from build123d import *

# Parameters (mm, degrees)
SKETCH_1_W          = 13
SKETCH_1_H          = 26
EXTRUDE_1_DEPTH     = 5.57372
SKETCH_2_W          = 13
SKETCH_2_H          = 3
EXTRUDE_2_DEPTH     = 9.8
SKETCH_4_R          = 1
CUT_EXTRUDE_1_DEPTH = 14
CHAMFER_2_SIZE      = 0.8
CHAMFER_2_SIZE2     = 1.385640646
SKETCH_5_R          = 1
EXTRUDE_3_DEPTH     = 13
SKETCH_6_R          = 1
CUT_EXTRUDE_2_DEPTH = 14


with BuildPart() as part:
    # ｽｹｯﾁ1 → ﾎﾞｽ - 押し出し1 (new body)
    with BuildSketch(Plane(origin=(0, 0, 0), x_dir=(1, 0, 0), z_dir=(0, 1, 0))):
        with Locations((6.5, 13)):
            Rectangle(SKETCH_1_W, SKETCH_1_H)
    extrude(amount=EXTRUDE_1_DEPTH)

    # ｽｹｯﾁ2 → ﾎﾞｽ - 押し出し2 (add)
    with BuildSketch(Plane(origin=(0, 5.57372, 0), x_dir=(1, 0, 0), z_dir=(0, 1, 0))):
        with Locations((6.5, 1.5)):
            Rectangle(SKETCH_2_W, SKETCH_2_H)
    extrude(amount=EXTRUDE_2_DEPTH)

    # ｽｹｯﾁ4 → ｶｯﾄ - 押し出し1 (cut, through all)
    with BuildSketch(Plane.ZY):
        with Locations((-16, 2.78686)):
            Circle(SKETCH_4_R)
        with Locations((-4, 2.78686)):
            Circle(SKETCH_4_R)
    extrude(amount=-CUT_EXTRUDE_1_DEPTH, mode=Mode.SUBTRACT)

    # 面取り2
    chamfer_2_edges = [part.edges().sort_by_distance(p)[0] for p in [
        (13, 0, -13),
        (0, 0, -13),
    ]]
    chamfer_2_side = [part.faces().sort_by_distance(p)[0] for p in [
        (6.5, 0, -13),
    ]]
    chamfer(chamfer_2_edges, length=CHAMFER_2_SIZE, length2=CHAMFER_2_SIZE2, reference=chamfer_2_side[0])

    # ｽｹｯﾁ5 → ﾎﾞｽ - 押し出し3 (add, through all)
    with BuildSketch(Plane.ZY):
        with Locations((-4, 2.78686)):
            Circle(SKETCH_5_R)
    extrude(amount=-EXTRUDE_3_DEPTH)

    # ｽｹｯﾁ6 → ｶｯﾄ - 押し出し2 (cut, through all)
    with BuildSketch(Plane.ZY):
        with Locations((-3.92837, 2.78686)):
            Circle(SKETCH_6_R)
    extrude(amount=-CUT_EXTRUDE_2_DEPTH, mode=Mode.SUBTRACT)


solid = part.part
CAD build for the part. Positions are in the model's coordinates, mm. A direction names the side the tool comes from. Round coordinates to 2 decimals unless told otherwise and drop trailing zeros. Order: outer loops, then holes, each group sorted by start corner. A loop starts at its lowest first (then second) coordinate and runs counter-clockwise, first axis right, second up. Notation, with made-up numbers: (58.25, -11) -> (78.25, -11) arc R20 ccw to (78.25, 18) -> close; hole circle Ø7 at (2.5, -13.5). An arc over 180 degrees is marked (long way). Write item = value, one per line. Start each with the question number.
(1) Cut at B-B, the plane y = 2.5. List the corners of the cut face in (x, z), then the cut area to 3 significant figures.
(2) Which spindle directions (+Z, -Z, +X, -X, +Y, -Y) get a long thin tool onto all of the face, cutting with end or side? Do faces 5 (the flat face through (13, 5, -10)), 6 (the flat face through (6, 5.574, -15)). Say none if no direction does.
(3) Pin check, flat tips, straight feed: P1, Ø1.8, axis at y = 2.79, z = -3.93, coming from the +X side; P2, Ø3, axis at x = 9, y = 11.5, coming from the -Z side; P3, Ø6.5, axis at x = 9.5, z = -14.5, coming from the +Y side; P4, Ø1.5, axis at x = 3, y = 8.5, coming from the +Z side. Stop position of each tip, or through.
(4) Cut at A-A, the plane z = -16. List the corners of the cut face in (x, y), then the cut area to 3 significant figures.
(5) Cut at D-D, the plane y = 9.5. List the corners of the cut face in (x, z).
(6) Probe line 1 (Y direction, x = 9, z = -16); line 2 (Z direction, x = 12.5, y = 3.5); line 3 (Z direction, x = 1.75, y = 11.5). List the from-to ranges inside material, lowest first. Write a range as [from, to].
(7) Cut at C-C, the plane x = 7.75. List the corners of the cut face in (y, z).
(8) Pull direction Y, two halves, no side cores. Call faces 1 (the flat face through (6, 0, -13)), 2 (the cylindrical face through (6.409, 3.087, -15.046)), 3 (the cylindrical face through (6.409, 3.087, -2.975)), 4 (the flat face through (6, 10, -3)): released by +Y, released by -Y, zero draft, split by the parting line, or undercut.
Model answer:
q1.outline = (0, -26) -> (13, -26) -> (13, -16.96) -> (0, -16.96) -> close; (0, -15.04) -> (13, -15.04) -> (13, -4.89) -> (0, -4.89) -> close; (0, -2.97) -> (13, -2.97) -> (13, 0) -> (0, 0) -> close
q1.area = 288 mm2
q2.face_5 = +Z, -Z, +X, +Y, -Y
q2.face_6 = -Z, +X, -X, +Y
q3.P1 = through
q3.P2 = -3
q3.P3 = 5.57
q3.P4 = 0
q4.outline = (0, 1.39) -> (0.8, 0) -> (12.2, 0) -> (13, 1.39) -> (13, 1.79) -> (0, 1.79) -> close; (0, 3.79) -> (13, 3.79) -> (13, 5.57) -> (0, 5.57) -> close
q4.area = 45.3 mm2
q5.outline = (0, -3) -> (13, -3) -> (13, 0) -> (0, 0) -> close
q6.line_1 = [0, 1.79], [3.79, 5.57]
q6.line_2 = [-26, -16.7], [-15.3, -4.63], [-3.23, 0]
q6.line_3 = [-3, 0]
q7.outline = (0, -26) -> (5.57, -26) -> (5.57, -3) -> (15.37, -3) -> (15.37, 0) -> (0, 0) -> close; hole circle Ø2 at (2.79, -16); hole circle Ø2 at (2.79, -3.93)
q8.face_1 = released by -Y
q8.face_2 = undercut
q8.face_3 = undercut
q8.face_4 = zero draft
